The model under review builds one solid part; all positions refer to its coordinate system, in mm. A direction names the side the tool comes from. Give positions to 0.01 mm unless a question says otherwise; leave off trailing zeros. Order: outer loops, then holes, each group sorted by start corner. A loop starts at its lowest first (then second) coordinate and runs counter-clockwise, first axis right, second up. Notation, with made-up numbers: (-5, 20) - (17, 20) arc R30 cw to (17, 47) - close; hole circle Ø5 at (80, 24.5). An arc over 180 degrees is marked (long way). Use CSV: the item, a comma, the result in double quotes. Start each with the question number.
1. For pin 1 (2.5 mm diameter, centred on x = 104.17, y = 43.38, fed in from +Z); pin 2 (1 mm diameter, centred on x = 108.5, z = -28.5, fed in from -Y); pin 3 (4 mm diameter, centred on x = 117, z = -28.5, fed in from -Y); pin 4 (4 mm diameter, centred on x = 122.5, z = -39, fed in from -Y), all flat-tipped, find the tip position at first contact; note any pin that passes through.
2. Take a section at B-B, the plane y = 38. State the section outline as (x, z) points, then the cut area to 3 significant figures.
3. Take a section at A-A, the plane z = -28.5. State the section outline as (x, y) points, then the cut area to 3 significant figures.
4. Take a section at C-C, the plane x = 99. State the section outline as (y, z) points, then the cut area to 3 significant figures.
5. Take a section at D-D, the plane y = 80.5. State the section outline as (x, z) points, then the cut area to 3 significant figures.
6. To check wall thickness, follow line 1 (Z direction, x = 117.5, y = 85.5); line 2 (X direction, y = 39, z = -41.5); line 3 (Y direction, x = 111, z = -32.25). State the ranges of each line that lie inside material, in increasing order. Write a range as [from, to].
7. Machinability: for faces 1 (the flat face through (102.11, 50.08, -30.59)), 2 (the flat face through (111.219, 41.453, -30.588)), 3 (the flat face through (98.2, 37.2, -30.6)), 4 (the flat face through (115.12, 54.35, -30.59)), which of the approach directions +Z, -Z, +X, -X, +Y, -Y give a long, thin tool a straight path to every point of the face, cutting with its end or side? Answer none if there is none.
```python
from build123d import *

# Parameters (mm, degrees)
BOSS_EXTRUDE1_DEPTH = 16
SKETCH3_R           = 1.65
CUT_EXTRUDE1_DEPTH  = 27
SKETCH4_R           = 80
BOSS_EXTRUDE2_DEPTH = 5
SKETCH5_R           = 1.65
CUT_EXTRUDE3_DEPTH  = 5


with BuildPart() as part:
    # Sketch2 → Boss-Extrude1 (new body)
    with BuildSketch(Plane(origin=(0, 0, -22.7), x_dir=(-1, 0, 0), z_dir=(0, 0, -1))):
        Polygon((-119.618145114, 49.851633515), (-102.581939837, 32.815428238), (-93.714762751, 41.682605324), (-110.750968028, 58.718810601), align=None)
    extrude(amount=BOSS_EXTRUDE1_DEPTH)

    # Sketch3 → Cut-Extrude1 (cut)
    with BuildSketch(Plane(origin=(0, 0, -22.7), x_dir=(-1, 0, 0), z_dir=(0, 0, -1))):
        with Locations(Location((-111.238929757, 50.452674279, 0), (0, 0, 180))):
            Circle(SKETCH3_R)
        with Locations(Location((-104.167861945, 43.381606467, 0), (0, 0, 180))):
            Circle(SKETCH3_R)
    extrude(amount=CUT_EXTRUDE1_DEPTH, mode=Mode.SUBTRACT)

    # Sketch4 → Boss-Extrude2 (add)
    with BuildSketch(Plane(origin=(0, 0, -38.7), x_dir=(-1, 0, 0), z_dir=(0, 0, -1))):
        with Locations((-111.238929757, 50.452674279)):
            Circle(SKETCH4_R)
    extrude(amount=BOSS_EXTRUDE2_DEPTH)

    # Sketch5 → Cut-Extrude3 (cut)
    with BuildSketch(Plane(origin=(0, 0, -38.7), x_dir=(-1, 0, 0), z_dir=(0, 0, -1))):
        with Locations((-111.238929757, 50.452674279)):
            Circle(SKETCH5_R)
        with Locations((-104.167861945, 43.381606467)):
            Circle(SKETCH5_R)
    extrude(amount=CUT_EXTRUDE3_DEPTH, mode=Mode.SUBTRACT)


solid = part.part
```
Determined:
1,pin 1,"passes through"
1,pin 2,"stops at y = 38.23"
1,pin 3,"stops at y = 45.23"
1,pin 4,"stops at y = -29.01"
2,outline,"(32.21, -43.7) - (190.26, -43.7) - (190.26, -38.7) - (107.77, -38.7) - (107.77, -22.7) - (97.4, -22.7) - (97.4, -38.7) - (32.21, -38.7) - close"
2,area,"956 mm²"
3,outline,"(93.71, 41.68) - (102.58, 32.82) - (119.62, 49.85) - (110.75, 58.72) - close; hole circle Ø3.3 at (104.17, 43.38); hole circle Ø3.3 at (111.24, 50.45)"
3,area,"285 mm²"
4,outline,"(-28.61, -43.7) - (129.51, -43.7) - (129.51, -38.7) - (46.97, -38.7) - (46.97, -22.7) - (36.4, -22.7) - (36.4, -38.7) - (-28.61, -38.7) - close"
4,area,"960 mm²"
5,outline,"(37.1, -43.7) - (185.38, -43.7) - (185.38, -38.7) - (37.1, -38.7) - close"
5,area,"741 mm²"
6,line 1,"z = [-43.7, -38.7]"
6,line 2,"x = [32.06, 190.41]"
6,line 3,"y = [41.23, 48.82], [52.09, 58.47]"
7,face 1,"+Z, -X, +Y"
7,face 2,"+Z, +X, -Y"
7,face 3,"+Z, -X, -Y"
7,face 4,"+Z, +X, +Y"
